```python
from build123d import *

# Parameters (mm, degrees)
SKETCH1_W           = 127.9906
SKETCH1_H           = 127.8382
BOSS_EXTRUDE1_DEPTH = 6.35
SKETCH3_R           = 2.54
SKETCH3_W           = 12.8016
SKETCH3_H           = 27.94
SKETCH3_W_2         = 18.034
SKETCH3_H_2         = 12.7
CUT_EXTRUDE1_DEPTH  = 7.35
SKETCH8_R           = 0.635
CUT_EXTRUDE2_DEPTH  = 20.05


with BuildPart() as part:
    # Sketch1 → Boss-Extrude1 (new body)
    with BuildSketch(Plane(origin=(0, 0, 0), x_dir=(1, 0, 0), z_dir=(0, 1, 0))):
        with Locations((63.9953, 63.9191)):
            Rectangle(SKETCH1_W, SKETCH1_H)
    extrude(amount=BOSS_EXTRUDE1_DEPTH)

    # Sketch3 → Cut-Extrude1 (cut, through all)
    with BuildSketch(Plane(origin=(0, 0, 0), x_dir=(-1, 0, 0), z_dir=(0, -1, 0))):
        with Locations((-63.9953, 25.4)):
            Circle(SKETCH3_R)
        with Locations((-63.9953, 102.4382)):
            Circle(SKETCH3_R)
        with BuildLine():
            Line((-5.08, 107.5182), (-11.43, 107.5182))
            ThreePointArc((-11.43, 107.5182), (-12.7, 108.7882), (-11.43, 110.0582))
            Line((-11.43, 110.0582), (-5.08, 110.0582))
            ThreePointArc((-5.08, 110.0582), (-3.81, 108.7882), (-5.08, 107.5182))
        make_face()
        with BuildLine():
            Line((-122.9106, 107.5182), (-116.5606, 107.5182))
            ThreePointArc((-116.5606, 107.5182), (-115.2906, 108.7882), (-116.5606, 110.0582))
            Line((-116.5606, 110.0582), (-122.9106, 110.0582))
            ThreePointArc((-122.9106, 110.0582), (-124.1806, 108.7882), (-122.9106, 107.5182))
        make_face()
        with BuildLine():
            Line((-122.9106, 20.32), (-116.5606, 20.32))
            ThreePointArc((-116.5606, 20.32), (-115.2906, 19.05), (-116.5606, 17.78))
            Line((-116.5606, 17.78), (-122.9106, 17.78))
            ThreePointArc((-122.9106, 17.78), (-124.1806, 19.05), (-122.9106, 20.32))
        make_face()
        with BuildLine():
            Line((-5.08, 20.32), (-11.43, 20.32))
            ThreePointArc((-11.43, 20.32), (-12.7, 19.05), (-11.43, 17.78))
            Line((-11.43, 17.78), (-5.08, 17.78))
            ThreePointArc((-5.08, 17.78), (-3.81, 19.05), (-5.08, 20.32))
        make_face()
        with BuildLine():
            Line((-20.32, 117.2083), (-26.67, 117.2083))
            ThreePointArc((-26.67, 117.2083), (-28.1813, 118.7196), (-26.67, 120.2309))
            Line((-26.67, 120.2309), (-20.32, 120.2309))
            ThreePointArc((-20.32, 120.2309), (-18.8087, 118.7196), (-20.32, 117.2083))
        make_face()
        with BuildLine():
            Line((-102.9081, 7.6073), (-106.0831, 7.6073))
            ThreePointArc((-106.0831, 7.6073), (-107.5944, 9.1186), (-106.0831, 10.6299))
            Line((-106.0831, 10.6299), (-102.9081, 10.6299))
            ThreePointArc((-102.9081, 10.6299), (-101.3968, 9.1186), (-102.9081, 7.6073))
        make_face()
        with Locations((-110.5154, 65.9384)):
            Rectangle(SKETCH3_W, SKETCH3_H)
        with Locations((-17.4752, 65.9384)):
            Rectangle(SKETCH3_W, SKETCH3_H)
        with Locations((-42.291, 73.4822)):
            Rectangle(SKETCH3_W_2, SKETCH3_H_2)
    extrude(amount=-CUT_EXTRUDE1_DEPTH, mode=Mode.SUBTRACT)

    # Sketch8 → Cut-Extrude2 (cut, through all)
    with BuildSketch(Plane.XZ.offset(12.7)):
        with Locations((19.05, -26.2382)):
            Circle(SKETCH8_R)
        with Locations((19.05, -13.5382)):
            Circle(SKETCH8_R)
        with Locations((19.05, -102.4382)):
            Circle(SKETCH8_R)
        with Locations((19.05, -115.1382)):
            Circle(SKETCH8_R)
        with Locations((57.15, -84.6582)):
            Circle(SKETCH8_R)
        with Locations((57.15, -46.5582)):
            Circle(SKETCH8_R)
        with Locations((96.2406, -46.5582)):
            Circle(SKETCH8_R)
        with Locations((96.2406, -84.6582)):
            Circle(SKETCH8_R)
        with Locations((107.95, -115.1382)):
            Circle(SKETCH8_R)
        with Locations((107.95, -102.4382)):
            Circle(SKETCH8_R)
        with Locations((107.95, -26.2382)):
            Circle(SKETCH8_R)
        with Locations((107.95, -13.5382)):
            Circle(SKETCH8_R)
    extrude(amount=-CUT_EXTRUDE2_DEPTH, mode=Mode.SUBTRACT)


solid = part.part
```
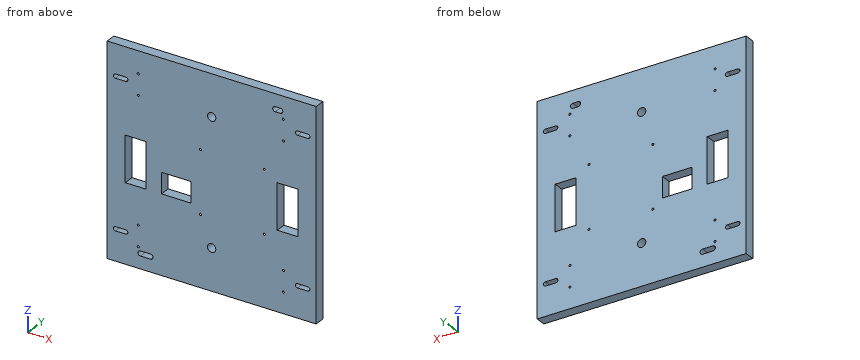
Geometry check sheet. Reference: the model listing, model coordinates, mm. Round coordinates to 2 decimals unless told otherwise and drop trailing zeros. Order: outer loops, then holes, each group sorted by start corner. A loop starts at its lowest first (then second) coordinate and runs counter-clockwise, first axis right, second up. Notation, with made-up numbers: (60, -11.5) - (99, -11.5) arc R18 ccw to (99, 7.5) - close; hole circle Ø3 at (-5, 84.25). An arc over 180 degrees is marked (long way). Use a Markdown table: item, result. Add a question column.
(1) Material ranges on line 1 along Z through (x, y) = (104.5, 6.25); line 2 along X through (y, z) = (0.5, -56.5); line 3 along Z through (x, y) = (107.95, 2.75), recorded low to high. Write a range as [from, to].
(2) Depth check by flat-ended pin: pin 1 (2 mm diameter, centred on y = 1, z = -82, fed in from -X); pin 2 (4.5 mm diameter, centred on x = 64, z = -102.44, fed in from +Y). Enter the tip coordinate at first touch or a pass-through.
(3) Sectioned sample at B-B, the plane y = 2.75. Count the separate pieces of the cut face and the enclosed holes in it, and give its area (3 significant figures).
(4) Sectioned sample at A-A, the plane z = -62. Enter the section's corners in (x, y), and give its area (3 significant figures).
Answers below:
| question | item | result |
|---|---|---|
| 1 | line 1 | [-127.84, -79.91], [-51.97, -10.63], [-7.61, 0] |
| 1 | line 2 | [0, 11.07], [23.88, 104.11], [116.92, 127.99] |
| 1 | line 3 | [-127.84, -115.77], [-114.5, -103.07], [-101.8, -79.91], [-51.97, -26.87], [-25.6, -14.17], [-12.9, 0] |
| 2 | pin 1 | x = 0 |
| 2 | pin 2 | through |
| 3 | separate pieces | 1 |
| 3 | enclosed holes | 23 |
| 3 | area | 15,200 mm² |
| 4 | outline | (0, 0) - (11.07, 0) - (11.07, 6.35) - (0, 6.35) - close; (23.88, 0) - (104.11, 0) - (104.11, 6.35) - (23.88, 6.35) - close; (116.92, 0) - (127.99, 0) - (127.99, 6.35) - (116.92, 6.35) - close |
| 4 | area | 650 mm² |
